from build123d import *

# Parameters (mm, degrees)
SKETCH_1_W                  = 230
SKETCH_1_H                  = 214.25
SKETCH_1_W_2                = 176
SKETCH_1_H_2                = 160.25
EXTRUDE_1_DEPTH             = 3
FILLET_1_R                  = 5
HOLE_WIZARD_6_4_6_4_1_D     = 6.4
HOLE_WIZARD_6_4_6_4_1_DEPTH = 3


with BuildPart() as part:
    # 草图1 → 凸台-拉伸1 (new body)
    with BuildSketch(Plane.XY):
        Rectangle(SKETCH_1_W, SKETCH_1_H)
        Rectangle(SKETCH_1_W_2, SKETCH_1_H_2, mode=Mode.SUBTRACT)
    extrude(amount=EXTRUDE_1_DEPTH)

    # 圆角1
    fillet_1_edges = [part.edges().sort_by_distance(p)[0] for p in [
        (-88, 80.125, 1.5),
        (-88, -80.125, 1.5),
        (88, -80.125, 1.5),
        (88, 80.125, 1.5),
        (-115, 107.125, 1.5),
        (115, 107.125, 1.5),
        (115, -107.125, 1.5),
        (-115, -107.125, 1.5),
    ]]
    fillet(fillet_1_edges, radius=FILLET_1_R)

    # Ø6.4 (6.4) 直径孔1
    with Locations(Plane.XY.offset(3)):
        with Locations((-95, 87.125), (95, 87.125), (95, -87.125), (-95, -87.125)):
            Hole(HOLE_WIZARD_6_4_6_4_1_D / 2, depth=HOLE_WIZARD_6_4_6_4_1_DEPTH)


solid = part.part
Here's how the part is built. I have some questions about the finished solid (model axes, mm). A direction names the side the tool comes from. Round coordinates to 2 decimals unless told otherwise and drop trailing zeros. Loops run counter-clockwise (first coordinate to the right, second up) from the corner with the lowest first, then second, coordinate; pieces in that order, holes last.
1. We'd pull the mould along X, two halves only. Please class faces 1 (the face through (-2, -94, 0)), 2 (the face through (-86.496, 78.699, 1.521)), 3 (the face through (113.496, 105.699, 1.521)): +X half, -X half, draft (parallel to the pull), parting line (faces both ways), or undercut.
Answer list:
face 1: draft
face 2: undercut
face 3: +X half
2. If we section it at B-B on y = 45: Write out the boundary of the cut face in (x, z), plus the area to 3 significant figures.
Answer list:
outline: (-115, 0) - (-88, 0) - (-88, 3) - (-115, 3) - close; (88, 0) - (115, 0) - (115, 3) - (88, 3) - close
area: 162 mm2
3. Which directions (+Z, -Z, +X, -X, +Y, -Y) give clear straight access to the entire face, cutting with the end or side of a thin tool? Please do faces 4 (the face through (-113.574, -105.621, 1.521)), 5 (the face through (86.574, 78.621, 1.521)).
Answer list:
face 4: +Z, -Z, -X, -Y
face 5: +Z, -Z
4. If I drill on line 1 along Y through (x, z) = (-95, 1.55) (3 decimals); line 2 along X through (y, z) = (-63.5, 1.25); line 3 along Y through (x, z) = (58, 2.75) (3 decimals), over which ranges is the centre line in solid material (lowest first)?
Answer list:
line 1: y = -107.125 to -90.325, -83.925 to 83.925, 90.325 to 107.125
line 2: x = -115 to -88, 88 to 115
line 3: y = -107.125 to -80.125, 80.125 to 107.125
5. If we section it at A-A on x = -95: Write out the boundary of the cut face in (y, z) (3 decimals), plus the area to 3 significant figures.
Answer list:
outline: (-107.125, 0) - (-90.325, 0) - (-90.325, 3) - (-107.125, 3) - close; (-83.925, 0) - (83.925, 0) - (83.925, 3) - (-83.925, 3) - close; (90.325, 0) - (107.125, 0) - (107.125, 3) - (90.325, 3) - close
area: 604 mm2
6. If we section it at D-D on x = 55.5: Write out the boundary of the cut face in (y, z) (3 decimals), plus the area to 3 significant figures.
Answer list:
outline: (-107.125, 0) - (-80.125, 0) - (-80.125, 3) - (-107.125, 3) - close; (80.125, 0) - (107.125, 0) - (107.125, 3) - (80.125, 3) - close
area: 162 mm2
7. If we section it at C-C on z = 0.6: Write out the boundary of the cut face in (x, y) (3 decimals).
Answer list:
outline: (-115, -102.125) arc R5 ccw to (-110, -107.125) - (110, -107.125) arc R5 ccw to (115, -102.125) - (115, 102.125) arc R5 ccw to (110, 107.125) - (-110, 107.125) arc R5 ccw to (-115, 102.125) - close; hole circle Ø6.4 at (-95, -87.125); hole circle Ø6.4 at (-95, 87.125); hole (-88, -75.125) arc R5 ccw to (-83, -80.125) - (83, -80.125) arc R5 ccw to (88, -75.125) - (88, 75.125) arc R5 ccw to (83, 80.125) - (-83, 80.125) arc R5 ccw to (-88, 75.125) - close; hole circle Ø6.4 at (95, -87.125); hole circle Ø6.4 at (95, 87.125)
